Autodesk Inventor part; units mm, degrees
ref_plane "YZ Plane" through (0, 0, 0) normal (1, 0, 0) x (0, 1, 0)
ref_plane "XZ Plane" through (0, 0, 0) normal (0, 1, 0) x (-1, 0, 0)
ref_plane "XY Plane" through (0, 0, 0) normal (0, 0, 1) x (1, 0, 0)
sketch "Sketch1" plane through (0, 0, 0) normal (0, 0, 1) x (1, 0, 0)
  arc A0 (-3, 3) -> (0, 0) centre (0, 3) ccw construction
  line L0 (0, 0) -> (121, 0) construction
  arc A1 (121, 0) -> (124, 3) centre (121, 3) ccw construction
  line L1 (124, 3) -> (124, 85) construction
  arc A2 (124, 85) -> (121, 88) centre (121, 85) ccw construction
  line L2 (121, 88) -> (0, 88) construction
  arc A3 (0, 88) -> (-3, 85) centre (0, 85) ccw construction
  line L3 (-3, 85) -> (-3, 3) construction
  arc A4 (63.75, 4.5) -> (63.75, 7.5) centre (63.75, 6) ccw construction
  line L4 (57.25, 4.5) -> (63.75, 4.5) construction
  arc A5 (57.25, 7.5) -> (57.25, 4.5) centre (57.25, 6) ccw construction
  line L5 (63.75, 7.5) -> (57.25, 7.5) construction
  arc A6 (70.5, 11.18) -> (70.5, 16.18) centre (70.5, 13.68) ccw construction
  line L6 (50.5, 11.18) -> (70.5, 11.18) construction
  arc A7 (50.5, 16.18) -> (50.5, 11.18) centre (50.5, 13.68) ccw construction
  line L7 (70.5, 16.18) -> (50.5, 16.18) construction
  arc A8 (43.75, 80.5) -> (43.75, 83.5) centre (43.75, 82) ccw construction
  line L8 (37.25, 80.5) -> (43.75, 80.5) construction
  arc A9 (37.25, 83.5) -> (37.25, 80.5) centre (37.25, 82) ccw construction
  line L9 (43.75, 83.5) -> (37.25, 83.5) construction
  arc A10 (70.5, 71.82) -> (70.5, 76.82) centre (70.5, 74.32) ccw construction
  line L10 (50.5, 71.82) -> (70.5, 71.82) construction
  arc A11 (50.5, 76.82) -> (50.5, 71.82) centre (50.5, 74.32) ccw construction
  line L11 (70.5, 76.82) -> (50.5, 76.82) construction
  circle A12 centre (30.65, 13.68) radius 3.55 construction
  circle A13 centre (10.65, 23.68) radius 2.55 construction
  circle A14 centre (30.65, 23.68) radius 2.55
  circle A15 centre (50.81, 23.68) radius 2.55
  circle A16 centre (80.35, 23.68) radius 2.55 construction
  circle A17 centre (100.35, 23.68) radius 2.55 construction
  circle A18 centre (100.35, 13.68) radius 2.55 construction
  circle A19 centre (80.35, 44) radius 2.55 construction
  circle A20 centre (90.35, 44) radius 2.55 construction
  circle A21 centre (80.35, 13.68) radius 2.55 construction
  circle A22 centre (100.35, 64.32) radius 2.55 construction
  circle A23 centre (80.35, 74.32) radius 2.55 construction
  circle A24 centre (90.35, 74.32) radius 2.55 construction
  circle A25 centre (30.65, 74.32) radius 3.55 construction
  circle A26 centre (40.18, 34) radius 2.55 construction
  circle A27 centre (30.65, 44) radius 3.55 construction
  circle A28 centre (70.19, 64.32) radius 2.55 construction
  circle A29 centre (20.65, 44) radius 3.55 construction
  circle A30 centre (60.5, 34) radius 2.55 construction
  circle A31 centre (100.35, 74.32) radius 2.55 construction
  circle A32 centre (90.82, 34) radius 2.55 construction
  circle A33 centre (110.35, 74.32) radius 2.55 construction
  circle A34 centre (90.82, 54) radius 2.55 construction
  circle A35 centre (75.325, 58.825) radius 2.55 construction
  circle A36 centre (30.65, 64.32) radius 2.55 construction
  circle A37 centre (10.65, 64.32) radius 2.55 construction
  circle A38 centre (45.675, 58.825) radius 2.55 construction
  circle A39 centre (10.65, 13.68) radius 3.55 construction
  circle A40 centre (10.65, 74.32) radius 3.55 construction
  circle A41 centre (50.5, 44) radius 2.55 construction
  circle A42 centre (60.5, 54) radius 2.55 construction
  circle A43 centre (60.5, 44) radius 2.55 construction
  circle A44 centre (70.5, 44) radius 2.55 construction
  circle A45 centre (40.18, 54) radius 2.55 construction
  circle A46 centre (10.65, 44) radius 3.55 construction
  circle A47 centre (30.18, 54) radius 2.55 construction
  circle A48 centre (60.5, 64.32) radius 2.55 construction
  circle A49 centre (20.65, 64.32) radius 2.55 construction
  circle A50 centre (20.65, 74.32) radius 3.55 construction
  circle A51 centre (80.82, 54) radius 2.55 construction
  circle A52 centre (40.65, 64.32) radius 2.55 construction
  circle A53 centre (110.35, 44) radius 2.55 construction
  circle A54 centre (110.35, 13.68) radius 2.55 construction
  circle A55 centre (80.82, 34) radius 2.55 construction
  circle A56 centre (75.325, 29.175) radius 2.55 construction
  circle A57 centre (50.81, 64.32) radius 2.55 construction
  circle A58 centre (80.35, 64.32) radius 2.55 construction
  circle A59 centre (45.675, 29.175) radius 2.55 construction
  circle A60 centre (30.18, 34) radius 2.55 construction
  circle A61 centre (40.65, 74.32) radius 3.55 construction
  circle A62 centre (40.65, 44) radius 3.55 construction
  circle A63 centre (90.35, 64.32) radius 2.55 construction
  circle A64 centre (110.35, 64.32) radius 2.55 construction
  circle A65 centre (100.35, 44) radius 2.55 construction
  circle A66 centre (60.5, 23.68) radius 2.55 construction
  circle A67 centre (90.35, 13.68) radius 2.55 construction
  circle A68 centre (110.35, 23.68) radius 2.55 construction
  circle A69 centre (90.35, 23.68) radius 2.55
  circle A70 centre (70.19, 23.68) radius 2.55
  circle A71 centre (40.65, 23.68) radius 2.55 construction
  circle A72 centre (20.65, 23.68) radius 2.55 construction
  circle A73 centre (40.65, 13.68) radius 3.55 construction
  circle A74 centre (20.65, 13.68) radius 3.55 construction
  arc A75 (63.75, 80.5) -> (63.75, 83.5) centre (63.75, 82) ccw construction
  line L12 (57.25, 80.5) -> (63.75, 80.5) construction
  arc A76 (57.25, 83.5) -> (57.25, 80.5) centre (57.25, 82) ccw construction
  line L13 (63.75, 83.5) -> (57.25, 83.5) construction
  arc A77 (77.25, 83.5) -> (77.25, 80.5) centre (77.25, 82) ccw construction
  line L14 (83.75, 83.5) -> (77.25, 83.5) construction
  arc A78 (83.75, 80.5) -> (83.75, 83.5) centre (83.75, 82) ccw construction
  line L15 (77.25, 80.5) -> (83.75, 80.5) construction
  arc A79 (43.75, 4.5) -> (43.75, 7.5) centre (43.75, 6) ccw construction
  line L16 (37.25, 4.5) -> (43.75, 4.5) construction
  arc A80 (37.25, 7.5) -> (37.25, 4.5) centre (37.25, 6) ccw construction
  line L17 (43.75, 7.5) -> (37.25, 7.5) construction
  arc A81 (77.25, 7.5) -> (77.25, 4.5) centre (77.25, 6) ccw construction
  line L18 (83.75, 7.5) -> (77.25, 7.5) construction
  arc A82 (83.75, 4.5) -> (83.75, 7.5) centre (83.75, 6) ccw construction
  line L19 (77.25, 4.5) -> (83.75, 4.5) construction
  line L20 (30.65, 23.68) -> (90.35, 23.68) construction
  line L21 (30.65, 11.18) -> (90.35, 11.18)
  line L22 (90.35, 36.18) -> (30.65, 36.18)
  arc A83 (30.65, 36.18) -> (30.65, 11.18) centre (30.65, 23.68) ccw
  arc A84 (90.35, 11.18) -> (90.35, 36.18) centre (90.35, 23.68) ccw
  line L23 (23.3543, 33.83) -> (97.6457, 33.83)
  line L24 (23.3543, 13.53) -> (97.6457, 13.53)
  point P0 (60.5, 23.68)
  dimension "d0" = 25
  dimension "d3" = 20.3
extrude "Extrusion1" add sketch "Sketch1" along normal blind 4
extrude "Extrusion2" add sketch "Sketch1" along normal blind 6 contours A83 L24 A84 L21 | A83 L22 A84 L23
sketch "Sketch2" plane through (30.65, 36.18, 0) normal (0, 1, 0) x (1, 0, 0)
  line L0 (0, -6) -> (59.7, -6)
  line L1 (29.85, -6) -> (29.85, 29.1247)
  point P0 (-30.65, 0)
surface extrude "ExtrusionSrf1" sketch "Sketch2" against normal blind 39.35 shown yes curves L1
properties part number "Espaciador Actuador - Antenas" material "PET Plastic"
Can you work these out from the model? Positions are in its coordinate system, mm. A direction names the side the tool comes from. Give positions to 0.01 mm unless a question says otherwise; leave off trailing zeros. Write each loop counter-clockwise with the first axis right and the second up, starting at its lowest first coordinate (ties: lowest second). Pieces come first, ordered by that corner, then holes. Notation, with made-up numbers: (61.25, 41.25) -> (67.25, 41.25) arc R6 cw to (67.25, 47.25) -> close; hole circle Ø8 at (57, 67). An arc over 180 degrees is marked (long way). One line per item, written item: value.
Q1. For P1, Ø6, axis at x = 30.65, y = 23.68, coming from the +Z side; P2, Ø3, axis at y = 14, z = 2.5, coming from the +X side, each with a flat end and sliding along its axis, tell me the tip position at first contact or that it passes through.
Results found:
P1: stops at z = 4
P2: stops at x = 99.8
Q2. Imagine slicing it at A-A on x = 50.81. Please give me the cut outline in (y, z).
Results found:
outline: (11.18, 0) -> (21.13, 0) -> (21.13, 4) -> (13.53, 4) -> (13.53, 6) -> (11.18, 6) -> close; (26.23, 0) -> (36.18, 0) -> (36.18, 6) -> (33.83, 6) -> (33.83, 4) -> (26.23, 4) -> close
Q3. Please list where these lines run through material, in increasing order: line 1 (Y direction, x = 90.35, z = 3.1); line 2 (X direction, y = 21.75, z = 3.6); line 3 (Z direction, x = 77, y = 23.75). Write a range as [from, to].
Results found:
line 1: y = [11.18, 21.13], [26.23, 36.18]
line 2: x = [18.3, 28.98], [32.32, 49.14], [52.48, 68.52], [71.86, 88.68], [92.02, 102.7]
line 3: z = [0, 4]
Q4. Imagine slicing it at B-B on y = 23.68. Please give me the cut outline in (x, z), and give its area (3 significant figures).
Results found:
outline: (18.15, 0) -> (28.1, 0) -> (28.1, 4) -> (18.15, 4) -> close; (33.2, 0) -> (48.26, 0) -> (48.26, 4) -> (33.2, 4) -> close; (53.36, 0) -> (67.64, 0) -> (67.64, 4) -> (53.36, 4) -> close; (72.74, 0) -> (87.8, 0) -> (87.8, 4) -> (72.74, 4) -> close; (92.9, 0) -> (102.85, 0) -> (102.85, 4) -> (92.9, 4) -> close
area: 257 mm^2
Q5. Imagine slicing it at C-C on z = 2.2. Please give me the cut outline in (x, y), and give its area (3 significant figures).
Results found:
outline: (30.65, 11.18) -> (90.35, 11.18) arc R12.5 ccw to (90.35, 36.18) -> (30.65, 36.18) arc R12.5 ccw to start; hole circle Ø5.1 at (30.65, 23.68); hole circle Ø5.1 at (50.81, 23.68); hole circle Ø5.1 at (70.19, 23.68); hole circle Ø5.1 at (90.35, 23.68)
area: 1,900 mm^2
Q6. Imagine slicing it at D-D on x = 87. Please give me the cut outline in (y, z), and give its area (3 significant figures).
Results found:
outline: (11.18, 0) -> (36.18, 0) -> (36.18, 6) -> (33.83, 6) -> (33.83, 4) -> (13.53, 4) -> (13.53, 6) -> (11.18, 6) -> close
area: 109 mm^2
Q7. We'd pull the mould along X, two halves only. Please class faces 1 (the face through (102.847, 23.955, 2.291)), 2 (the face through (53.166, 24.657, 1.972)), 3 (the face through (60, 13.53, 5)): +X half, -X half, draft (parallel to the pull), parting line (faces both ways), or undercut.
Results found:
face 1: +X half
face 2: undercut
face 3: draft
Q8. Which directions (+Z, -Z, +X, -X, +Y, -Y) give clear straight access to the entire face, cutting with the end or side of a thin tool? Please do faces 4 (the face through (60, 33.83, 5)), 5 (the face through (60, 24, 0)).
Results found:
face 4: +Z, +X, -X
face 5: -Z, +X, -X, +Y, -Y
